Read the model definition and answer for the solid it produces. Units are mm, in the model's axes. Face numbers are marked on the shaded views. A direction names the side the tool comes from. Coordinates: 2 decimals unless noted, no trailing zeros. Write each loop counter-clockwise with the first axis right and the second up, starting at its lowest first coordinate (ties: lowest second). Pieces come first, ordered by that corner, then holes. Notation, with made-up numbers: (5.25, 60) - (31.25, 60) arc R17 ccw to (31.25, 89) - close; hole circle Ø7 at (-39.5, 38). An arc over 180 degrees is marked (long way). Return JSON: item names as keys, results as strings.
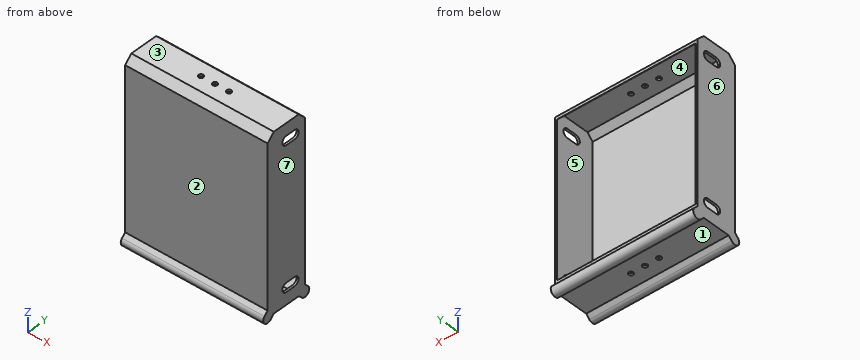
```python
from build123d import *

# Parameters (mm, degrees)
SKETCH1_W                                = 203.2
SKETCH1_H                                = 247.65
BOSS_EXTRUDE1_DEPTH                      = 60
CHAMFER1_SIZE                            = 10
SHELL3_T                                 = -3
CUT_EXTRUDE1_REACH                       = 247.403
MIRROR1_AT_THE_SECOND_PLANE_COPY_1_REACH = 247.403
CUT_EXTRUDE2_REACH                       = 276.323
SKETCH3_R                                = 3.45
BOSS_EXTRUDE2_DEPTH                      = 203.2


with BuildPart() as part:
    # Sketch1 → Boss-Extrude1 (new body)
    with BuildSketch(Plane(origin=(0, 0, 0), x_dir=(1, 0, 0), z_dir=(0, 1, 0))):
        Rectangle(SKETCH1_W, SKETCH1_H)
    extrude(amount=BOSS_EXTRUDE1_DEPTH)

    # Chamfer1
    chamfer1_edges = [part.edges().sort_by_distance(p)[0] for p in [
        (0, 60, 123.825),
        (0, 0, 123.825),
        (0, 0, -123.825),
        (0, 60, -123.825),
    ]]
    chamfer(chamfer1_edges, length=CHAMFER1_SIZE)

    # Shell3
    shell3_openings = [part.faces().sort_by_distance(p)[0] for p in [
        (0, 60, 0),
    ]]
    offset(amount=SHELL3_T, openings=shell3_openings, kind=Kind.INTERSECTION)

    # Sketch2 → Cut-Extrude1 (cut, up to next)
    with BuildSketch(Plane.ZY.offset(101.6), mode=Mode.PRIVATE) as cut_extrude1_sk1:
        with BuildLine():
            Line((-93.675, 43.55), (-93.675, 30))
            ThreePointArc((-93.675, 30), (-100.025, 23.65), (-106.375, 30))
            Line((-106.375, 30), (-106.375, 43.55))
            ThreePointArc((-106.375, 43.55), (-100.025, 49.9), (-93.675, 43.55))
        make_face()
    cut_extrude1_tool1 = extrude(cut_extrude1_sk1.sketch, amount=-CUT_EXTRUDE1_REACH, mode=Mode.PRIVATE) & part.part
    cut_extrude1 = cut_extrude1_tool1.solids().sort_by_distance((-101.6, 36.775, -100.025))[0]
    add(cut_extrude1, mode=Mode.SUBTRACT)

    # Mirror1: Cut-Extrude1 across plane
    add(cut_extrude1.mirror(Plane.XY), mode=Mode.SUBTRACT)

    # Mirror1 at the second plane: Cut-Extrude1 across plane
    add(cut_extrude1.mirror(Plane(origin=(0, 0, 0), x_dir=(0, 0, 1), z_dir=(1, 0, 0))), mode=Mode.SUBTRACT)

    # Mirror1 at the second plane copy 1 sketc → Mirror1 at the second plane copy 1 (cut, up to next)
    with BuildSketch(Plane(origin=(101.6, 0, 0), x_dir=(0, 0, -1), z_dir=(1, 0, 0)), mode=Mode.PRIVATE) as mirror1_at_the_second_plane_copy_1_sk1:
        with BuildLine():
            Line((-93.675, 43.55), (-93.675, 30))
            ThreePointArc((-93.675, 30), (-100.025, 23.65), (-106.375, 30))
            Line((-106.375, 30), (-106.375, 43.55))
            ThreePointArc((-106.375, 43.55), (-100.025, 49.9), (-93.675, 43.55))
        make_face()
    mirror1_at_the_second_plane_copy_1_tool1 = extrude(mirror1_at_the_second_plane_copy_1_sk1.sketch, amount=-MIRROR1_AT_THE_SECOND_PLANE_COPY_1_REACH, mode=Mode.PRIVATE) & part.part
    add(mirror1_at_the_second_plane_copy_1_tool1.solids().sort_by_distance((101.6, 36.775, 100.025))[0], mode=Mode.SUBTRACT)

    # Sketch3 → Cut-Extrude2 (cut, up to next)
    with BuildSketch(Plane(origin=(0, 0, -123.825), x_dir=(-1, 0, 0), z_dir=(0, 0, -1)), mode=Mode.PRIVATE) as cut_extrude2_sk1:
        with Locations((0, 30)):
            Circle(SKETCH3_R)
    cut_extrude2_tool1 = extrude(cut_extrude2_sk1.sketch, amount=-CUT_EXTRUDE2_REACH, mode=Mode.PRIVATE) & part.part
    # Sketch3 → Cut-Extrude2 (cut, up to next)
    with BuildSketch(Plane(origin=(0, 0, -123.825), x_dir=(-1, 0, 0), z_dir=(0, 0, -1)), mode=Mode.PRIVATE) as cut_extrude2_sk2:
        with Locations((20, 30)):
            Circle(SKETCH3_R)
    cut_extrude2_tool2 = extrude(cut_extrude2_sk2.sketch, amount=-CUT_EXTRUDE2_REACH, mode=Mode.PRIVATE) & part.part
    # Sketch3 → Cut-Extrude2 (cut, up to next)
    with BuildSketch(Plane(origin=(0, 0, -123.825), x_dir=(-1, 0, 0), z_dir=(0, 0, -1)), mode=Mode.PRIVATE) as cut_extrude2_sk3:
        with Locations((-20, 30)):
            Circle(SKETCH3_R)
    cut_extrude2_tool3 = extrude(cut_extrude2_sk3.sketch, amount=-CUT_EXTRUDE2_REACH, mode=Mode.PRIVATE) & part.part
    cut_extrude2_1 = cut_extrude2_tool1.solids().sort_by_distance((0, 30, -123.825))[0]
    add(cut_extrude2_1, mode=Mode.SUBTRACT)
    cut_extrude2_2 = cut_extrude2_tool2.solids().sort_by_distance((-20, 30, -123.825))[0]
    add(cut_extrude2_2, mode=Mode.SUBTRACT)
    cut_extrude2_3 = cut_extrude2_tool3.solids().sort_by_distance((20, 30, -123.825))[0]
    add(cut_extrude2_3, mode=Mode.SUBTRACT)
    cut_extrude2 = cut_extrude2_1 + cut_extrude2_2 + cut_extrude2_3  # Cut-Extrude2 as one shape, for the pattern or mirror that repeats it

    # Mirror2: Cut-Extrude2 across plane
    add(cut_extrude2.mirror(Plane.XY), mode=Mode.SUBTRACT)

    # Sketch4 → Boss-Extrude2 (add)
    with BuildSketch(Plane.ZY.offset(101.6)):
        with BuildLine():
            Line((-123.825, 50), (-128.825, 55))
            ThreePointArc((-128.825, 55), (-128.825, 65), (-118.825, 65))
            Line((-118.825, 65), (-113.825, 60))
            Line((-113.825, 60), (-123.825, 50))
        make_face()
        with BuildLine():
            Line((-123.825, 10), (-113.825, 0))
            Line((-113.825, 0), (-118.825, -5))
            ThreePointArc((-118.825, -5), (-128.825, -5), (-128.825, 5))
            Line((-128.825, 5), (-123.825, 10))
        make_face()
    extrude(amount=-BOSS_EXTRUDE2_DEPTH)


solid = part.part
```
(1) A cutting plane is placed at B-B (y = 15.5). Determine the outline of the cut face in (x, z) (3 decimals).
Answer:
{"outline": "(-101.6, -123.825) - (101.6, -123.825) - (101.6, 123.825) - (-101.6, 123.825) - close; hole (-98.6, -120.825) - (98.6, -120.825) - (98.6, 120.825) - (-98.6, 120.825) - close"}
(2) A cutting plane is placed at D-D (x = 87.5). Determine the outline of the cut face in (y, z) (3 decimals).
Answer:
{"outline": "(-5, -118.825) arc R7.071 ccw to (5, -128.825) - (10, -123.825) - (50, -123.825) - (55, -128.825) arc R7.071 ccw to (65, -118.825) - (60, -113.825) - (60, -109.582) - (48.757, -120.825) - (11.243, -120.825) - (3, -112.582) - (3, 112.582) - (11.243, 120.825) - (48.757, 120.825) - (60, 109.582) - (60, 113.825) - (50, 123.825) - (10, 123.825) - (0, 113.825) - (0, -113.825) - close"}
(3) Which of the six approach directions +Z, -Z, +X, -X, +Y, -Y give full straight-line access (tool end or side, diameter ignored) to the marked faces 1, 2, 3 and 4?
Answer:
{"face 1": "-Z, +X, -X", "face 2": "+Z, +X, -X, -Y", "face 3": "+Z, +X, -X, +Y, -Y", "face 4": "none"}
(4) A cutting plane is placed at A-A (x = -20). Determine the outline of the cut face in (y, z) (3 decimals).
Answer:
{"outline": "(-5, -118.825) arc R7.071 ccw to (5, -128.825) - (10, -123.825) - (26.55, -123.825) - (26.55, -120.825) - (11.243, -120.825) - (3, -112.582) - (3, 112.582) - (11.243, 120.825) - (26.55, 120.825) - (26.55, 123.825) - (10, 123.825) - (0, 113.825) - (0, -113.825) - close; (33.45, -123.825) - (50, -123.825) - (55, -128.825) arc R7.071 ccw to (65, -118.825) - (60, -113.825) - (60, -109.582) - (48.757, -120.825) - (33.45, -120.825) - close; (33.45, 120.825) - (48.757, 120.825) - (60, 109.582) - (60, 113.825) - (50, 123.825) - (33.45, 123.825) - close"}
(5) Straight lines are drawn through the part: line 1 (Z direction, x = 41, y = 44) (3 decimals); line 2 (Y direction, x = 20, z = -122.9); line 3 (X direction, y = 13.5, z = 37.5). For each, find the intervals that lie inside material, in ascending order. Write a range as from..to.
Answer:
{"line 1": "-123.825..-120.825, 120.825..123.825", "line 2": "-7.01..26.55, 33.45..67.01", "line 3": "-101.6..-98.6, 98.6..101.6"}
(6) A cutting plane is placed at C-C (z = 73). Determine the outline of the cut face in (x, y).
Answer:
{"outline": "(-101.6, 0) - (101.6, 0) - (101.6, 60) - (98.6, 60) - (98.6, 3) - (-98.6, 3) - (-98.6, 60) - (-101.6, 60) - close"}
(7) Determine the mould class of the marked faces 5, 6 and 7 for opening direction X: +X half, -X half, draft (parallel to the pull), parting line (faces both ways), or undercut.
Answer:
{"face 5": "undercut", "face 6": "-X half", "face 7": "+X half"}
(8) Flat-ended cylindrical pins translate along their axes: P1, Ø4, axis at x = 50, z = 21.5, coming from the +Y side; P2, Ø4, axis at x = 63, y = 3.5, coming from the +Z side (3 decimals); P3, Ø1, axis at x = 29, z = -45, coming from the -Y side. Find the tip coordinate at first contact, or state that the pin passes through.
Answer:
{"P1": "y = 3", "P2": "z = 119.325", "P3": "y = 0"}
